Source: CAD feature listing. Evaluate the final solid. Frame: model axes, mm. A direction names the side the tool comes from. Coordinates: 2 decimals unless noted, no trailing zeros. Write each loop counter-clockwise with the first axis right and the second up, starting at its lowest first coordinate (ties: lowest second). Pieces come first, ordered by that corner, then holes. Notation, with made-up numbers: (24, -3) -> (46, -3) arc R15 ccw to (46, 10) -> close; hole circle Ø3 at (70, 46). An arc over 180 degrees is marked (long way). One line per item, written item: value. Start each with the question number.
1. First-contact query: P1, Ø2.5, axis at x = 129.75, y = 37.3, coming from the +Z side; P2, Ø1.6, axis at y = 47.5, z = 123.5, coming from the +X side; P3, Ø1.6, axis at y = 48, z = 128.5, coming from the -X side; P4, Ø10, axis at x = 57, z = 69, coming from the +Y side. Flat tips, straight axial feed; report the tip coordinate or a pass-through.
2. Access query for faces 1 (the flat face through (126, 23, 110)), 2 (the flat face through (8, 44, 110)), 3 (the flat face through (68, 0, 110)). Directions: +Z, -Z, +X, -X, +Y, -Y. A direction counts if a zero-diameter tool reaches every point of the face in a straight line with its end or side. Return the directions, or none.
3. Section query A-A, the plane z = 125. Output: boundary loops of the cut face in (x, y), and give its area (3 significant figures).
4. Section query C-C, the plane x = 55.5. Output: boundary loops of the cut face in (y, z), and give its area (3 significant figures).
5. Section query B-B, the plane y = 6.5. Output: boundary loops of the cut face in (x, z).
6. Mould query, pull axis X, two halves, no side actions, for faces 4 (the flat face through (7, 47, 110)), 5 (the flat face through (137, 24, 110)), 6 (the flat face through (0, 25, 110)). Classes: released by +X, released by -X, zero draft, split by the parting line, or undercut.
7. Line query: line 1 (Y direction, x = 129.75, z = 116); line 2 (X direction, y = 37.5, z = 171.5); line 3 (X direction, y = 4.5, z = 73). Output: solid intervals per line, ascending.
from build123d import *

# Parameters (mm, degrees)
SKETCH_R     = 2.05
PAD_DEPTH    = 223.52
CHAMFER_SIZE = 4


with BuildPart() as part:
    # Sketch → Pad (new body)
    with BuildSketch(Plane.XY):
        Polygon((0, 0), (137, 0), (137, 49), (127, 49), (127, 47), (133, 47), (133, 44), (126, 44), (126, 2), (11, 2), (11, 44), (4, 44), (4, 47), (10, 47), (10, 49), (0, 49), align=None)
        with Locations((7.25, 11.7)):
            Circle(SKETCH_R, mode=Mode.SUBTRACT)
        with Locations((129.75, 11.7)):
            Circle(SKETCH_R, mode=Mode.SUBTRACT)
        with Locations((7.25, 37.3)):
            Circle(SKETCH_R, mode=Mode.SUBTRACT)
        with Locations((129.75, 37.3)):
            Circle(SKETCH_R, mode=Mode.SUBTRACT)
    extrude(amount=PAD_DEPTH)

    # Chamfer
    chamfer_edges = [part.edges().sort_by_distance(p)[0] for p in [
        (0, 49, 111.76),
        (137, 49, 111.76),
        (137, 0, 111.76),
        (0, 0, 111.76),
    ]]
    chamfer(chamfer_edges, length=CHAMFER_SIZE)


solid = part.part
Computed values:
1. P1: passes through
1. P2: stops at x = 135.3
1. P3: stops at x = 2.2
1. P4: stops at y = 2
2. face 1: +Z, -Z, +Y
2. face 2: +Z, -Z
2. face 3: +Z, -Z, +X, -X, -Y
3. outline: (0, 4) -> (4, 0) -> (133, 0) -> (137, 4) -> (137, 45) -> (133, 49) -> (127, 49) -> (127, 47) -> (133, 47) -> (133, 44) -> (126, 44) -> (126, 2) -> (11, 2) -> (11, 44) -> (4, 44) -> (4, 47) -> (10, 47) -> (10, 49) -> (4, 49) -> (0, 45) -> close; hole circle Ø4.1 at (7.25, 11.7); hole circle Ø4.1 at (7.25, 37.3); hole circle Ø4.1 at (129.75, 11.7); hole circle Ø4.1 at (129.75, 37.3)
3. area: 1,180 mm²
4. outline: (0, 0) -> (2, 0) -> (2, 223.52) -> (0, 223.52) -> close
4. area: 447 mm²
5. outline: (0, 0) -> (11, 0) -> (11, 223.52) -> (0, 223.52) -> close; (126, 0) -> (137, 0) -> (137, 223.52) -> (126, 223.52) -> close
6. face 4: undercut
6. face 5: released by +X
6. face 6: released by -X
7. line 1: y = 0 to 9.65, 13.75 to 35.25, 39.35 to 44, 47 to 49
7. line 2: x = 0 to 5.21, 9.29 to 11, 126 to 127.71, 131.79 to 137
7. line 3: x = 0 to 11, 126 to 137
